from build123d import *

# Parameters (mm, degrees)
BOSS_EXTRUDE1_DEPTH = 31.75
SKETCH2_W           = 38.1
SKETCH2_H           = 25.4
CUT_EXTRUDE1_DEPTH  = 27.94
SKETCH3_R           = 3.175
BOSS_EXTRUDE2_DEPTH = 25.4
SKETCH5_R           = 1.905
CUT_EXTRUDE2_DEPTH  = 32.75


with BuildPart() as part:
    # Sketch1 → Boss-Extrude1 (new body)
    with BuildSketch(Plane.XY):
        Polygon((0, 0), (-38.1, 0), (-38.1, 6.35), (-38.1, 27.94), (-31.75, 27.94), (-31.75, 19.05), (0, 19.05), align=None)
    extrude(amount=BOSS_EXTRUDE1_DEPTH)

    # Sketch2 → Cut-Extrude1 (cut)
    with BuildSketch(Plane(origin=(0, 27.94, 0), x_dir=(1, 0, 0), z_dir=(0, 1, 0))):
        with Locations((-19.05, -15.875)):
            Rectangle(SKETCH2_W, SKETCH2_H)
    extrude(amount=-CUT_EXTRUDE1_DEPTH, mode=Mode.SUBTRACT)

    # Sketch3 → Boss-Extrude2 (add)
    with BuildSketch(Plane.XY.offset(3.175)):
        with Locations((-31.75, 12.446)):
            Circle(SKETCH3_R)
    extrude(amount=BOSS_EXTRUDE2_DEPTH)

    # Sketch5 → Cut-Extrude2 (cut, through all)
    with BuildSketch(Plane.XY.offset(31.75)):
        with Locations((-6.35, 12.7)):
            Circle(SKETCH5_R)
    extrude(amount=-CUT_EXTRUDE2_DEPTH, mode=Mode.SUBTRACT)


solid = part.part
Read the model definition and answer for the solid it produces. Units are mm, in the model's axes. A direction names the side the tool comes from. Coordinates: 2 decimals unless noted, no trailing zeros. Loops run counter-clockwise (first coordinate to the right, second up) from the corner with the lowest first, then second, coordinate; pieces in that order, holes last.
Q1. The part is cut by section C-C on x = -6.35. Write down the section's boundary in (y, z) (3 decimals).
Q2. The part is cut by section B-B on y = 19.75. Write down the section's boundary in (x, z) (3 decimals).
Q3. Each of these flat-tipped pins is pushed along its axis until it touches: pin 1 Ø1 at (y, z) = (21.5, 2) entering from +X; pin 2 Ø2.5 at (x, z) = (-11, 30) entering from +Y; pin 3 Ø10 at (y, z) = (14.5, 16.5) entering from -X (3 decimals). Where does it stop, or does it pass through?
Q4. The mould has two halves that part along X. Classify faces 1 (the face through (-19, 0, 2)), 2 (the face through (-31.75, 24, 2)), 3 (the face through (-7.86, 11.54, 1.61)): +X half, -X half, draft (parallel to the pull), parting line (faces both ways), or undercut.
Q5. The part is cut by section D-D on y = 11.5. Write down the section's boundary in (x, z) (3 decimals), and give its area (3 significant figures).
Q6. Which of the six approach directions +Z, -Z, +X, -X, +Y, -Y give full straight-line access (tool end or side, diameter ignored) to faces 4 (the face through (-19, 11, 31.75)), 5 (the face through (-31.75, 24, 30))?
Q7. Consider probe 1 along Y at (x, z) = (-6.35, 30.6) (3 decimals); probe 2 along Z at (x, y) = (-22, 18.25) (3 decimals); probe 3 along Y at (x, z) = (-24.5, 2.5). Determine where each line is inside the solid, lowest interval first.
Q8. The part is cut by section A-A on x = -25. Write down the section's boundary in (y, z) (3 decimals).
Results below:
1. outline: (0, 0) - (10.795, 0) - (10.795, 3.175) - (0, 3.175) - close; (0, 28.575) - (10.795, 28.575) - (10.795, 31.75) - (0, 31.75) - close; (14.605, 0) - (19.05, 0) - (19.05, 3.175) - (14.605, 3.175) - close; (14.605, 28.575) - (19.05, 28.575) - (19.05, 31.75) - (14.605, 31.75) - close
2. outline: (-38.1, 0) - (-31.75, 0) - (-31.75, 3.175) - (-38.1, 3.175) - close; (-38.1, 28.575) - (-31.75, 28.575) - (-31.75, 31.75) - (-38.1, 31.75) - close
3. pin 1: stops at x = -31.75
3. pin 2: stops at y = 19.05
3. pin 3: stops at x = -34.925
4. face 1: draft
4. face 2: +X half
4. face 3: undercut
5. outline: (-38.1, 0) - (-7.83, 0) - (-7.83, 3.175) - (-28.719, 3.175) - (-28.719, 28.575) - (-7.83, 28.575) - (-7.83, 31.75) - (-38.1, 31.75) - (-38.1, 28.575) - (-34.781, 28.575) - (-34.781, 3.175) - (-38.1, 3.175) - close; (-4.87, 0) - (0, 0) - (0, 3.175) - (-4.87, 3.175) - close; (-4.87, 28.575) - (0, 28.575) - (0, 31.75) - (-4.87, 31.75) - close
5. area: 377 mm2
6. face 4: +Z, +X, -X, +Y, -Y
6. face 5: +Z, -Z, +X, +Y
7. probe 1: y = 0 to 10.795, 14.605 to 19.05
7. probe 2: z = 0 to 3.175, 28.575 to 31.75
7. probe 3: y = 0 to 19.05
8. outline: (0, 0) - (19.05, 0) - (19.05, 3.175) - (0, 3.175) - close; (0, 28.575) - (19.05, 28.575) - (19.05, 31.75) - (0, 31.75) - close
